Source: CAD feature listing. Evaluate the final solid. Frame: model axes, mm. A direction names the side the tool comes from. Give positions to 0.01 mm unless a question says otherwise; leave off trailing zeros. Order: outer loops, then holes, each group sorted by start corner. A loop starts at its lowest first (then second) coordinate and runs counter-clockwise, first axis right, second up.
```python
from build123d import *


with BuildPart() as f1:
    # F0 (on Front) → F1 (revolve)
    with BuildSketch(Plane.XZ):
        with BuildLine():
            Line((32.216486, 72.812662), (0, 72.812662))
            Line((0, 72.812662), (0, -55.692833))
            Line((0, -55.692833), (30.984804, -55.692833))
            Line((30.984804, -55.692833), (30.984804, -45.839377))
            ThreePointArc((30.984804, -45.839377), (22.47862, -33.23833), (19.489104, -18.331811))
            Line((19.489104, -18.331811), (19.489104, 33.809394))
            ThreePointArc((19.489104, 33.809394), (22.372698, 50.087954), (32.216486, 63.369766))
            Line((32.216486, 63.369766), (32.216486, 72.812662))
        make_face()
    revolve(axis=Axis((0, 0, -0.267141), (0, 0, -1)))


solid = f1.part
```
1) Section query C-C, the plane z = 31.5. Return the cut outline in (x, y).
Report:
outline: circle Ø38.98 at (0, 0)
2) Section query A-A, the plane x = 0. Return the cut outline in (y, z), and give its area (3 significant figures).
Report:
outline: (-32.22, 63.37) arc R36.07 cw to (-19.49, 33.81) - (-19.49, -18.33) arc R38.66 cw to (-30.98, -45.84) - (-30.98, -55.69) - (30.98, -55.69) - (30.98, -45.84) arc R38.66 cw to (19.49, -18.33) - (19.49, 33.81) arc R36.07 cw to (32.22, 63.37) - (32.22, 72.81) - (-32.22, 72.81) - close
area: 5,880 mm2
3) Section query D-D, the plane z = 52.5. Return the cut outline in (x, y).
Report:
outline: circle Ø47.04 at (0, 0)
4) Material intervals for L1, parallel to Z at x = 18.5, y = -11; L2, parallel to Y at x = 14.5, z = -15.5; L3, parallel to Y at x = 1, z = -17.5, sorted ascending.
Report:
L1: z = -55.69 to -30.71, 47.93 to 72.81
L2: y = -13.02 to 13.02
L3: y = -19.46 to 19.46
5) Pin query (flat end, axial travel): pin 1 (12 mm diameter, centred on x = -24.5, z = -34, fed in from -Y); pin 2 (12 mm diameter, centred on y = 18, z = -18.5, fed in from +X); pin 3 (1 mm diameter, centred on x = 5.5, z = -28.5, fed in from +Y). Return the tip coordinate at first contact, or that it passes through.
Report:
pin 1: stops at y = -14.79
pin 2: stops at x = 15.36
pin 3: stops at y = 20.31
6) Reachability of faces 1 (the cylindrical face through (-4.03, -30.72, -50.7)), 2 (the cylindrical face through (-6.98, 31.45, 68.16)), 3 (the cylindrical face through (18.59, -5.85, 8.1)) from +Z, -Z, +X, -X, +Y, -Y: full face, straight path, thin tool, end or side. Return the list, or none.
Report:
face 1: -Z
face 2: +Z, -Z
face 3: none
